from build123d import *

# Parameters (mm, degrees)
SKETCH1_W           = 40.1
SKETCH1_H           = 10
BOSS_EXTRUDE1_DEPTH = 5
SKETCH2_W           = 40.1
SKETCH2_H           = 5
BOSS_EXTRUDE2_DEPTH = 37
BOSS_EXTRUDE3_DEPTH = 5
SKETCH4_R           = 1.2
SKETCH4_R_2         = 2.5
CUT_EXTRUDE1_DEPTH  = 38
SKETCH5_R           = 4.955
SKETCH5_R_2         = 2.5
CUT_EXTRUDE2_DEPTH  = 36


with BuildPart() as part:
    # Sketch1 → Boss-Extrude1 (new body)
    with BuildSketch(Plane.XY):
        with Locations((20.05, -5)):
            Rectangle(SKETCH1_W, SKETCH1_H)
        with BuildLine():
            ThreePointArc((8, -18), (19.970074906, -29.999962687), (31.999850748, -18.059850002))
            ThreePointArc((31.999850748, -18.059850002), (34.386559706, -12.358242505), (40.1, -10))
            Line((40.1, -10), (0, -10))
            ThreePointArc((0, -10), (5.656854249, -12.343145751), (8, -18))
        make_face()
    extrude(amount=BOSS_EXTRUDE1_DEPTH)

    # Sketch2 → Boss-Extrude2 (add)
    with BuildSketch(Plane.XY.offset(5)):
        with Locations((20.05, 2.5)):
            Rectangle(SKETCH2_W, SKETCH2_H)
    extrude(amount=-BOSS_EXTRUDE2_DEPTH)

    # Sketch3 → Boss-Extrude3 (add)
    with BuildSketch(Plane(origin=(0, 5, 0), x_dir=(1, 0, 0), z_dir=(0, 1, 0))):
        with BuildLine():
            Line((0, 32), (0, 0))
            ThreePointArc((0, 0), (-13.95, 16), (0, 32))
        make_face()
        with BuildLine():
            Line((40.1, 32), (40.1, 0))
            ThreePointArc((40.1, 0), (54.05, 16), (40.1, 32))
        make_face()
    extrude(amount=-BOSS_EXTRUDE3_DEPTH)

    # Sketch4 → Cut-Extrude1 (cut, through all)
    with BuildSketch(Plane.XY.offset(5)):
        with Locations((20.012468828, -13)):
            Circle(SKETCH4_R)
        with Locations((20, -18)):
            Circle(SKETCH4_R_2)
        with Locations((15, -17.975062189)):
            Circle(SKETCH4_R)
        with Locations((19.987531172, -23)):
            Circle(SKETCH4_R)
        with Locations((25, -18.024937811)):
            Circle(SKETCH4_R)
    extrude(amount=-CUT_EXTRUDE1_DEPTH, mode=Mode.SUBTRACT)

    # Sketch5 → Cut-Extrude2 (cut, through all)
    with BuildSketch(Plane(origin=(0, 5, 0), x_dir=(1, 0, 0), z_dir=(0, 1, 0))):
        with Locations((31.88, 16)):
            Circle(SKETCH5_R)
        with Locations((-3.95, 16)):
            Circle(SKETCH5_R_2)
    extrude(amount=-CUT_EXTRUDE2_DEPTH, mode=Mode.SUBTRACT)


solid = part.part
Input: part model. Units: mm. Frame: model coordinates. A direction names the side the tool comes from. Coordinates: 2 decimals unless noted, no trailing zeros. Loops run counter-clockwise (first coordinate to the right, second up) from the corner with the lowest first, then second, coordinate; pieces in that order, holes last.
(1) Set-up query: faces 1 (the face through (0, -3, 3)), 2 (the face through (40.1, -3, 3)), 3 (the face through (20, -11, 0)), 4 (the face through (21, 5, -14)). Return all of +Z, -Z, +X, -X, +Y, -Y with unobstructed straight access to the full face (end or side cutting, diameter ignored); none if empty.
(2) Section D-D on z = -20. Return the cut outline in (x, y).
(3) Pull-direction query (Y, two-part tool) for faces 5 (the face through (5.594, -12.281, 2.465)), 6 (the face through (-13.947, 2.535, -15.676)), 7 (the face through (24.05, -18.76, 2.54)), 8 (the face through (19.06, -13.73, 2.54)); classes: released by +Y, released by -Y, zero draft, split by the parting line, or undercut.
(4) Section B-B on y = -13. Return the cut outline in (x, z) (3 decimals), then the cut area to 3 significant figures.
(5) Material intervals for probe 1 along Y at (x, z) = (20, 2); probe 2 along X at (y, z) = (1, -16) (3 decimals); probe 3 along X at (y, z) = (1.5, -15.5), sorted ascending.
(6) Section A-A on y = 2.5. Return the cut outline in (x, z) (3 decimals).
(7) First-contact query: pin 1 Ø16 at (x, z) = (31.88, -16) entering from -Y; pin 2 Ø3 at (x, y) = (1.5, -8.5) entering from -Z; pin 3 Ø1.5 at (y, z) = (-2, 3) entering from +X. Flat tips, straight axial feed; report the tip coordinate or a pass-through.
(8) Section C-C on x = 20. Return the cut outline in (y, z), then the cut area to 3 significant figures.
Data:
1. face 1: +Z, -X, +Y, -Y
1. face 2: +Z, +X, +Y, -Y
1. face 3: -Z, +X, -X, -Y
1. face 4: +Z, -Z, +X, -X, +Y
2. outline: (-13.45, 0) - (28.96, 0) - (28.96, 5) - (-13.45, 5) - close; (34.8, 0) - (53.55, 0) - (53.55, 5) - (34.8, 5) - close
3. face 5: released by -Y
3. face 6: zero draft
3. face 7: undercut
3. face 8: undercut
4. outline: (6.245, 0) - (18.812, 0) - (18.812, 5) - (6.245, 5) - close; (21.212, 0) - (33.807, 0) - (33.807, 5) - (21.212, 5) - close
4. area: 126 mm2
5. probe 1: y = -30 to -24.2, -21.8 to -20.5, -15.5 to -14.2, -11.8 to 5
5. probe 2: x = -13.95 to -6.45, -1.45 to 26.925, 36.835 to 54.05
5. probe 3: x = -13.94 to -6.4, -1.5 to 26.95, 36.81 to 54.04
6. outline: (0, -32) - (40.1, -32) arc R16.151 ccw to (40.1, 0) - (40.1, 5) - (0, 5) - (0, 0) arc R16.151 ccw to start; hole circle Ø5 at (-3.95, -16); hole circle Ø9.91 at (31.88, -16)
7. pin 1: stops at y = 0
7. pin 2: stops at z = 0
7. pin 3: stops at x = 40.1
8. outline: (-30, 0) - (-24.2, 0) - (-24.2, 5) - (-30, 5) - close; (-21.8, 0) - (-20.5, 0) - (-20.5, 5) - (-21.8, 5) - close; (-15.5, 0) - (-14.2, 0) - (-14.2, 5) - (-15.5, 5) - close; (-11.8, 0) - (0, 0) - (0, -32) - (5, -32) - (5, 5) - (-11.8, 5) - close
8. area: 286 mm2
